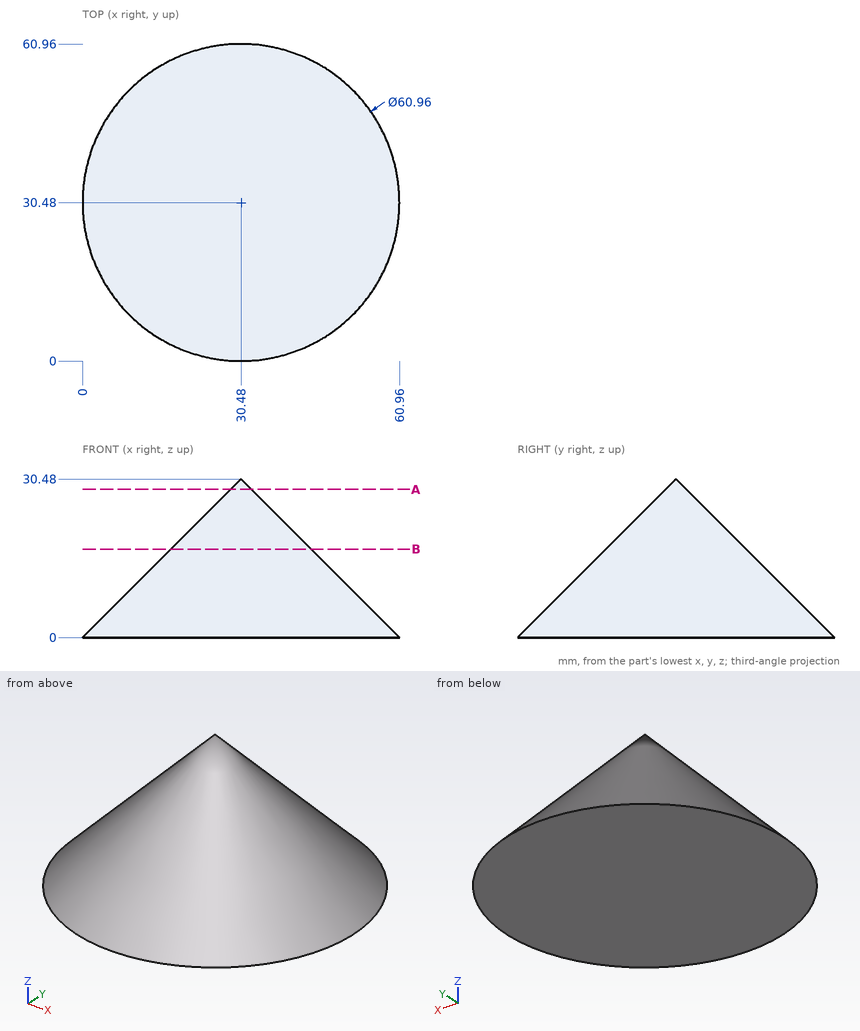
Input: dimensioned drawing with shaded views. Units: mm. Origin: part minimum x, y, z. Give positions to 0.01 mm unless a question says otherwise; leave off trailing zeros. Write each loop counter-clockwise with the first axis right and the second up, starting at its lowest first coordinate (ties: lowest second). Pieces come first, ordered by that corner, then holes.
Q1. First-contact query: P1, Ø12, axis at x = 27.5, z = 12.5, coming from the +Y side; P2, Ø1, axis at y = 47.5, z = 5.5, coming from the +X side; P3, Ø2, axis at x = 51, y = 10.5, coming from the +Z side. Flat tips, straight axial feed; report the tip coordinate or a pass-through.
Q2. Material intervals for probe 1 along Y at (x, z) = (33, 22.5); probe 2 along Z at (x, y) = (23.5, 58.5); probe 3 along Y at (x, z) = (21, 7), sorted ascending.
Q3. Section A-A, the plane z = 28.5. Output: boundary loops of the cut face in (x, y), plus the area to 3 significant figures.
Q4. Section B-B, the plane z = 17. Output: boundary loops of the cut face in (x, y).
Filled in:
1. P1: stops at y = 54.31
1. P2: stops at x = 49.58
1. P3: stops at z = 2.84
2. probe 1: y = 22.91 to 38.05
2. probe 2: z = 0 to 1.6
2. probe 3: y = 9 to 51.96
3. outline: circle Ø3.96 at (30.48, 30.48)
3. area: 12.3 mm2
4. outline: circle Ø26.96 at (30.48, 30.48)
